```python
from build123d import *

# Parameters (mm, degrees)
F0_W     = 76.2
F0_H     = 76.2
F1_DEPTH = 25.4
F2_DEPTH = 76.2
F3_W     = 25.4
F3_H     = 25.4
F4_DEPTH = 14.732


# Not quite as in the source:
# - the program builds the solid bodies; features that only make, move or delete a surface that nothing else refers to are left out


with BuildPart() as f1:
    # F0 (on Front) → F1 (new body)
    with BuildSketch(Plane.XZ):
        with Locations((-38.1, 42.3055109791)):
            Rectangle(F0_W, F0_H)
    extrude(amount=F1_DEPTH)

    # F0 (on Front) → F2 (join)
    with BuildSketch(Plane.XZ):
        with Locations((-38.1, 42.3055109791)):
            Rectangle(F0_W, F0_H)
    extrude(amount=F2_DEPTH)

    # F3 (on face) → F4 (join)
    with BuildSketch(Plane.XZ.offset(76.2)):
        with Locations((-38.1, 40.3138278052)):
            Rectangle(F3_W, F3_H)
    extrude(amount=F4_DEPTH)


solid = f1.part
```
Geometry check sheet. Reference: the model listing, model coordinates, mm. A direction names the side the tool comes from. Coordinates: 2 decimals unless noted, no trailing zeros. Order: outer loops, then holes, each group sorted by start corner. A loop starts at its lowest first (then second) coordinate and runs counter-clockwise, first axis right, second up.
Item 1: Section check B-B (z = 34). Enter the section's corners in (x, y).
Item 2: Section check D-D (x = -8). Enter the section's corners in (y, z), plus the area to 3 significant figures.
Item 3: Section check C-C (y = -77.5). Enter the section's corners in (x, z).
Item 4: Tool access check on faces 1 (the flat face through (-38, -83, 53.014)), 2 (the flat face through (-38, -83, 27.614)), 3 (the flat face through (-50.8, -83, 40)), 4 (the flat face through (-25.4, -83, 40)). Record the directions out of +Z, -Z, +X, -X, +Y, -Y that give a thin tool (end or side, any length) a straight path to the whole face; none if there is none.
Item 5: Section check A-A (x = -33.5). Enter the section's corners in (y, z), plus the area to 3 significant figures.
Item 6: Depth check by flat-ended pin: pin 1 (4.5 mm diameter, centred on x = -37.5, y = -82, fed in from +Z); pin 2 (4 mm diameter, centred on x = -37, z = 16.5, fed in from -Y); pin 3 (16 mm diameter, centred on y = -84.5, z = 46.5, fed in from -X). Enter the tip coordinate at first touch or a pass-through.
Item 7: Scan lines: line 1 along Y through (x, z) = (-17.5, 14.5); line 2 along Z through (x, y) = (-43, -81). Record each from-to range of solid material in increasing order.
Check sheet entries:
1. outline: (-76.2, -76.2) - (-50.8, -76.2) - (-50.8, -90.93) - (-25.4, -90.93) - (-25.4, -76.2) - (0, -76.2) - (0, 0) - (-76.2, 0) - close
2. outline: (-76.2, 4.21) - (0, 4.21) - (0, 80.41) - (-76.2, 80.41) - close
2. area: 5,810 mm2
3. outline: (-50.8, 27.61) - (-25.4, 27.61) - (-25.4, 53.01) - (-50.8, 53.01) - close
4. face 1: +Z, +X, -X, -Y
4. face 2: -Z, +X, -X, -Y
4. face 3: +Z, -Z, -X, -Y
4. face 4: +Z, -Z, +X, -Y
5. outline: (-90.93, 27.61) - (-76.2, 27.61) - (-76.2, 4.21) - (0, 4.21) - (0, 80.41) - (-76.2, 80.41) - (-76.2, 53.01) - (-90.93, 53.01) - close
5. area: 6,180 mm2
6. pin 1: stops at z = 53.01
6. pin 2: stops at y = -76.2
6. pin 3: stops at x = -50.8
7. line 1: y = -76.2 to 0
7. line 2: z = 27.61 to 53.01
